Part model, mm, in its own coordinate system. A direction names the side the tool comes from. Give positions to 0.01 mm unless a question says otherwise; leave off trailing zeros. Order: outer loops, then holes, each group sorted by start corner. A loop starts at its lowest first (then second) coordinate and runs counter-clockwise, first axis right, second up.
from build123d import *

# Parameters (mm, degrees)
F2_R     = 7.188692
F3_DEPTH = 127
F4_R     = 7.484689
F5_DEPTH = 25.4


with BuildPart() as f1:
    # F0 (on Front) → F1 (revolve)
    with BuildSketch(Plane.XZ):
        with BuildLine():
            Line((-27.215535, 0), (-17.227892, 0))
            Line((-17.227892, 0), (-17.227892, 34.93984))
            Line((-17.227892, 34.93984), (0, 34.93984))
            Line((0, 34.93984), (0, 41.325383))
            Line((0, 41.325383), (-19.68387, 41.325383))
            ThreePointArc((-19.68387, 41.325383), (-22.520971, 42.534607), (-23.613434, 45.418683))
            Line((-23.613434, 45.418683), (-27.215535, 45.418683))
            Line((-27.215535, 45.418683), (-27.215535, 33.466253))
            Line((-27.215535, 33.466253), (-24.104631, 33.466253))
            Line((-24.104631, 33.466253), (-24.104631, 30.519081))
            Line((-24.104631, 30.519081), (-27.215535, 30.519081))
            Line((-27.215535, 30.519081), (-27.215535, 29.350575))
            Line((-27.215535, 29.350575), (-23.940898, 29.350575))
            Line((-23.940898, 29.350575), (-23.940898, 27.878314))
            Line((-23.940898, 27.878314), (-27.215535, 27.878314))
            Line((-27.215535, 27.878314), (-27.215535, 26.098322))
            Line((-27.215535, 26.098322), (-23.940898, 26.098322))
            Line((-23.940898, 26.098322), (-23.940898, 22.709342))
            Line((-23.940898, 22.709342), (-27.215535, 22.709342))
            Line((-27.215535, 22.709342), (-27.215535, 0))
        make_face()
    revolve(axis=Axis((0, 0, 38.132612), (0, 0, -1)))

    # F2 (on Right) → F3 (cut)
    with BuildSketch(Plane.YZ):
        with Locations((0, 12.0396)):
            Circle(F2_R)
    extrude(amount=-F3_DEPTH, mode=Mode.SUBTRACT)

    # F4 (on Right) → F5 (cut)
    with BuildSketch(Plane.YZ):
        with Locations((0, 12.3444)):
            Circle(F4_R)
    extrude(amount=-F5_DEPTH, mode=Mode.SUBTRACT)


solid = f1.part
Item 1: Pull direction X, two halves, no side cores. Call faces 5 (the face through (0, 0, 41.325)), 6 (the face through (0.1, -24.1, 26.098)), 7 (the face through (-25.96, 8.17, 11.2)): released by +X, released by -X, zero draft, split by the parting line, or undercut.
Item 2: Band-saw the part on A-A on z = 15. List the corners of the cut face in (x, y), plus the area to 3 significant figures.
Item 3: Which spindle directions (+Z, -Z, +X, -X, +Y, -Y) get a long thin tool onto all of the face, cutting with end or side? Do faces 1 (the face through (-0.1, -24.1, 22.709)), 2 (the face through (0, 0, 34.94)), 3 (the face through (-18, 0, 0)), 4 (the face through (-24.766, 0.313, 4.858)). Say none if no direction does.
Item 4: Drill centre lines: probe 1 along Z at (x, y) = (-10, 24.5); probe 2 along Y at (x, z) = (0, 9.5); probe 3 along Z at (x, y) = (-23.75, 0). Where is each one in solid material? Low to high.
Item 5: Drop flat-ended pins along their axis: P1, Ø10, axis at x = -1, y = -9.5, coming from the -Z side; P2, Ø1.5, axis at x = 20, z = 9.5, coming from the -Y side; P3, Ø2, axis at x = -5, z = 35.5, coming from the +Y side. Give the stop position or say it passes through.
Working result:
1. face 5: undercut
1. face 6: zero draft
1. face 7: split by the parting line
2. outline: (-26.42, -6.55) arc R27.22 ccw (long way) to (-26.42, 6.55) - (-25.4, 6.55) - (-25.4, 7) - (-15.74, 7) arc R17.23 cw (long way) to (-15.74, -7) - (-25.4, -7) - (-25.4, -6.55) - close
2. area: 1,250 mm2
3. face 1: none
3. face 2: -Z
3. face 3: -Z, +X, -X, +Y, -Y
3. face 4: -X
4. probe 1: z = 0 to 22.71, 26.1 to 27.88, 29.35 to 30.52, 33.47 to 45.42
4. probe 2: y = -27.22 to -17.23, 17.23 to 27.22
4. probe 3: z = 0 to 4.85, 19.83 to 45.42
5. P1: stops at z = 34.94
5. P2: stops at y = -19.24
5. P3: stops at y = 26.92
